Work out the finished part from the listing and answer in its coordinate system (mm). A direction names the side the tool comes from. Round coordinates to 2 decimals unless told otherwise and drop trailing zeros. Order: outer loops, then holes, each group sorted by start corner. A loop starts at its lowest first (then second) coordinate and runs counter-clockwise, first axis right, second up. Notation, with made-up numbers: (66, -22.5) -> (78, -22.5) arc R17 ccw to (78, -15.5) -> close; hole circle Ø7 at (81, 88). An arc over 180 degrees is marked (long way). Use one line per item in the form item = value.
Autodesk Inventor part; units mm, degrees
ref_plane "YZ Plane" through (0, 0, 0) normal (1, 0, 0) x (0, 1, 0)
ref_plane "XZ Plane" through (0, 0, 0) normal (0, 1, 0) x (-1, 0, 0)
ref_plane "XY Plane" through (0, 0, 0) normal (0, 0, 1) x (1, 0, 0)
sketch "Sketch1" plane through (0, 0, 0) normal (0, 1, 0) x (-1, 0, 0)
  circle A0 centre (0, 0) radius 3.9
  dimension "d0" = 7.8
extrude "Extrusion1" add sketch "Sketch1" along normal blind 10
sketch "Sketch2" plane through (0, 10, 0) normal (0, 1, 0) x (1, 0, 0)
  circle A0 centre (0, 0) radius 7
  dimension "d3" = 14
extrude "Extrusion2" add sketch "Sketch2" along normal blind 2
chamfer "Chamfer1" distance 1 angle 45 1 edges at (-7, 12, 0)
properties part number "_3DPrint"
Item 1: The part is cut by section D-D, the plane y = 11.25. Give the vertices of the cut face in (x, z).
Findings:
outline = circle Ø13.5 at (0, 0)
Item 2: The part is cut by section C-C, the plane y = 2.25. Give the vertices of the cut face in (x, z).
Findings:
outline = circle Ø7.8 at (0, 0)
Item 3: Consider line 1 along Y through (x, z) = (3.75, 4.25); line 2 along Z through (x, y) = (0, 7.75); line 3 along Y through (x, z) = (6, -3). Determine where each line is inside the solid, lowest interval first.
Findings:
line_1 = 10 to 12
line_2 = -3.9 to 3.9
line_3 = 10 to 11.29
Item 4: The part is cut by section B-B, the plane x = 0. Give the vertices of the cut face in (y, z), and give its area (3 significant figures).
Findings:
outline = (0, -3.9) -> (10, -3.9) -> (10, -7) -> (11, -7) -> (12, -6) -> (12, 6) -> (11, 7) -> (10, 7) -> (10, 3.9) -> (0, 3.9) -> close
area = 105 mm^2
Item 5: The part is cut by section A-A, the plane z = 0. Give the vertices of the cut face in (x, y).
Findings:
outline = (-7, 10) -> (-3.9, 10) -> (-3.9, 0) -> (3.9, 0) -> (3.9, 10) -> (7, 10) -> (7, 11) -> (6, 12) -> (-6, 12) -> (-7, 11) -> close
Item 6: Flat-ended cylindrical pins translate along their axes: P1, Ø2, axis at x = -1, y = 3.5, coming from the +Z side; P2, Ø1, axis at y = 10.5, z = -2, coming from the +X side; P3, Ø1.5, axis at y = 5, z = -3, coming from the -X side. Find the tip coordinate at first contact, or state that the pin passes through.
Findings:
P1 = 3.9
P2 = 6.84
P3 = -3.19
Item 7: For faces 1 (the cylindrical face through (2.87, 4.93, -2.64)), 2 (the flat face through (0, 12, 0)), determine the directions among +Z, -Z, +X, -X, +Y, -Y from which every point of the face is accessible in a straight line to the end or side of a thin tool.
Findings:
face_1 = -Y
face_2 = +Z, -Z, +X, -X, +Y
